Autodesk Inventor part; units mm, degrees
ref_plane "Work Plane1" through (-7, 7, 9) normal (0, 1, 0) x (1, 0, 0)
ref_plane "YZ Plane" through (0, 0, 0) normal (1, 0, 0) x (0, 1, 0)
ref_plane "XZ Plane" through (0, 0, 0) normal (0, 1, 0) x (-1, 0, 0)
sketch "Sketch1" plane through (0, 0, 0) normal (0, 0, 1) x (1, 0, 0)
  circle A0 centre (0, 0) radius 7
  dimension "d0" = 14
extrude "Extrusion1" add sketch "Sketch1" along normal blind 9
ref_plane "Work Plane1" through (-7, 7, 9) normal (0, 1, 0) x (1, 0, 0)
sketch "Sketch3" plane through (-7, 7, 9) normal (0, 1, 0) x (1, 0, 0)
  circle A0 centre (7, 4.5) radius 1.2
  dimension "d9" = 2.4
hole "Hole1" at (0, 7, 4.5) direction (0, -1, 0) diameter 2.459 depth 7
sketch "Sketch4" plane through (0, 0, 0) normal (0, 0, -1) x (-1, 0, 0)
  circle A0 centre (0, 0) radius 7
  circle A1 centre (0, 0) radius 3.5
  dimension "d17" = 7
extrude "Extrusion3" add sketch "Sketch4" along normal blind 6 contours A1
properties part number "gear hridel"
Geometry check sheet. Reference: the model listing, model coordinates, mm. A direction names the side the tool comes from. Coordinates: 2 decimals unless noted, no trailing zeros. Order: outer loops, then holes, each group sorted by start corner. A loop starts at its lowest first (then second) coordinate and runs counter-clockwise, first axis right, second up. Notation, with made-up numbers: M 28,22.5 L 75,22.5 A14 ccw 75,43.5 Z; hole C 5.5,70.5 d3. An arc over 180 degrees is marked long. Use CSV: the item, a comma, the result in double quotes.
Item 1: Cross-section at D-D on z = -0.5. Record the cut outline in (x, y).
Returned:
outline,"C 0,0 d7"
Item 2: Thickness scan on line 1 along Z through (x, y) = (0, 3); line 2 along Z through (x, y) = (0, 4); line 3 along Z through (x, y) = (6, 0.25). Record the ranges inside material, lowest first.
Returned:
line 1,"z = -6 to 3.27, 5.73 to 9"
line 2,"z = 0 to 3.27, 5.73 to 9"
line 3,"z = 0 to 9"
Item 3: Cross-section at C-C on y = -0.75. Record the cut outline in (x, z), then the cut area to 3 significant figures.
Returned:
outline,"M -6.96,0 L -3.42,0 L -3.42,-6 L 3.42,-6 L 3.42,0 L 6.96,0 L 6.96,9 L -6.96,9 Z"
area,"166 mm2"
Item 4: Gauge pin test, flat ends, axial feed: pin 1 Ø2 at (y, z) = (-5.5, -4) entering from +X; pin 2 Ø0.7 at (x, z) = (0, 5) entering from +Y; pin 3 Ø3 at (x, z) = (-4, 6) entering from -Y; pin 4 Ø5 at (y, z) = (-4, -3.5) entering from +X. Record the tip position at first contact, or that the pin passes through.
Returned:
pin 1,"passes through"
pin 2,"stops at y = 0"
pin 3,"stops at y = -6.54"
pin 4,"stops at x = 3.16"
Item 5: Mould release check, pull along Z, two halves, no side actions. Record for faces 3 (the cylindrical face through (-3.233, 1.341, -2.958)), 4 (the flat face through (3, -3, 0)), 5 (the flat face through (0, 0, 9)), 6 (the cylindrical face through (-0.05, 3.45, 3.27)): pulls with the +Z half, pulls with the -Z half, needs draft (parallel to the pull), parting line crosses it, or undercut.
Returned:
face 3,"needs draft"
face 4,"pulls with the -Z half"
face 5,"pulls with the +Z half"
face 6,"undercut"
Item 6: Cross-section at B-B on y = 1.5. Record the cut outline in (x, z), then the cut area to 3 significant figures.
Returned:
outline,"M -6.84,0 L -3.16,0 L -3.16,-6 L 3.16,-6 L 3.16,0 L 6.84,0 L 6.84,9 L -6.84,9 Z; hole C 0,4.5 d2.46"
area,"156 mm2"
Item 7: Tool access check on faces 1 (the flat face through (0, 0, 4)), 2 (the flat face through (0, 0, -6)). Record the directions out of +Z, -Z, +X, -X, +Y, -Y that give a thin tool (end or side, any length) a straight path to the whole face; none if there is none.
Returned:
face 1,"+Y"
face 2,"-Z, +X, -X, +Y, -Y"
Item 8: Cross-section at A-A on x = 0. Record the cut outline in (y, z), then the cut area to 3 significant figures.
Returned:
outline,"M -7,0 L -3.5,0 L -3.5,-6 L 3.5,-6 L 3.5,0 L 7,0 L 7,3.27 L 0,3.27 L 0,5.73 L 7,5.73 L 7,9 L -7,9 Z"
area,"151 mm2"
